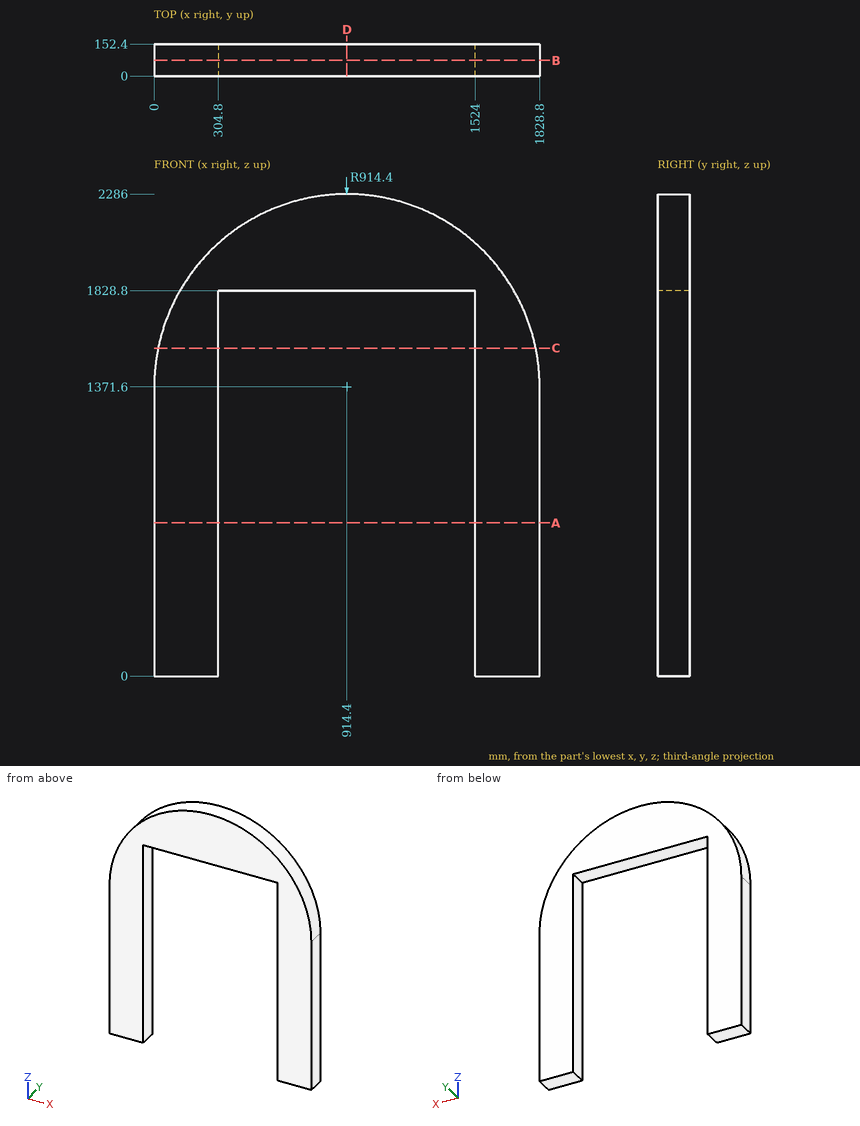
Drawing for the job (mm, zero at the part's lowest x, y, z). Coordinates: 2 decimals unless noted, no trailing zeros. Loops run counter-clockwise (first coordinate to the right, second up) from the corner with the lowest first, then second, coordinate; pieces in that order, holes last. Notation, with made-up numbers: (-13, -17) - (28, -17) arc R17 ccw to (28, 10) - close; hole circle Ø3 at (-39, 26.25). An arc over 180 degrees is marked (long way). Return JSON: item names as keys, results as strings.
1. Band-saw the part on C-C (z = 1556). Give the cut face in (x, y).
Result:
{"outline": "(18.79, 0) - (304.8, 0) - (304.8, 152.4) - (18.79, 152.4) - close; (1524, 0) - (1810.01, 0) - (1810.01, 152.4) - (1524, 152.4) - close"}
2. Drop flat-ended pins along their axis: pin 1 (8 mm diameter, centred on y = 115.5, z = 1432.5, fed in from +X); pin 2 (3 mm diameter, centred on y = 66, z = 1521, fed in from -X); pin 3 (4 mm diameter, centred on x = 626, y = 88.5, fed in from +Z). Give the stop position or say it passes through.
Result:
{"pin 1": "stops at x = 1827.03", "pin 2": "stops at x = 12.04", "pin 3": "stops at z = 2239.99"}
3. Band-saw the part on A-A (z = 726). Give the cut face in (x, y).
Result:
{"outline": "(0, 0) - (304.8, 0) - (304.8, 152.4) - (0, 152.4) - close; (1524, 0) - (1828.8, 0) - (1828.8, 152.4) - (1524, 152.4) - close"}
4. Band-saw the part on D-D (x = 914.4). Give the cut face in (y, z), and give its area (3 significant figures).
Result:
{"outline": "(0, 1828.8) - (152.4, 1828.8) - (152.4, 2286) - (0, 2286) - close", "area": "69,700 mm2"}
5. Band-saw the part on B-B (y = 75). Give the cut face in (x, z), and give its area (3 significant figures).
Result:
{"outline": "(0, 0) - (304.8, 0) - (304.8, 1828.8) - (1524, 1828.8) - (1524, 0) - (1828.8, 0) - (1828.8, 1371.6) arc R914.4 ccw to (0, 1371.6) - close", "area": "1,590,000 mm2"}
6. Probe L1, parallel to X at y = 132, z = 173; L2, parallel to X at y = 30, z = 1378; L3, parallel to Z at x = 650, y = 41.5. List the from-to ranges inside material, lowest first. Write a range as from..to.
Result:
{"L1": "x = 0..304.8, 1524..1828.8", "L2": "x = 0.02..304.8, 1524..1828.78", "L3": "z = 1828.8..2246.94"}
